from build123d import *

# Parameters (mm, degrees)
SKETCH1_R                = 1.75
BOSS_EXTRUDE1_DEPTH      = 3
BOSS_EXTRUDE2_DEPTH      = 15
BOSS_EXTRUDE3_REACH      = 34.671
BOSS_EXTRUDE3_END_RADIUS = 91.49157749
SKETCH4_R                = 1.75
CUT_EXTRUDE1_DEPTH       = 31.604747935


with BuildPart() as part:
    # Sketch1 → Boss-Extrude1 (new body)
    with BuildSketch(Plane.XY):
        with BuildLine():
            Line((0.117990197, 5), (14.645149272, 5))
            ThreePointArc((14.645149272, 5), (15.76191903, 15.092961754), (17.99029172, 25))
            Line((17.99029172, 25), (2.99029172, 25))
            ThreePointArc((2.99029172, 25), (1.076516113, 15.068594129), (0.117990197, 5))
        make_face()
        with Locations((3.988971184, 10)):
            Circle(SKETCH1_R, mode=Mode.SUBTRACT)
        with Locations((5.276368215, 19)):
            Circle(SKETCH1_R, mode=Mode.SUBTRACT)
    extrude(amount=BOSS_EXTRUDE1_DEPTH)

    # Sketch2 → Boss-Extrude2 (add)
    with BuildSketch(Plane.XY.offset(3)):
        with BuildLine():
            Line((0.117990197, 5), (14.645149272, 5))
            ThreePointArc((14.645149272, 5), (14.739672725, 6.500878193), (14.858852588, 8))
            Line((14.858852588, 8), (0.302317906, 8))
            ThreePointArc((0.302317906, 8), (0.199520295, 6.500653365), (0.117990197, 5))
        make_face()
    extrude(amount=BOSS_EXTRUDE2_DEPTH)

    # Boss-Extrude3: up to this cylinder (the profile starts outside it)
    boss_extrude3_end = Plane(origin=(106, 0, 8), z_dir=(0, 0, -1)) * Cylinder(BOSS_EXTRUDE3_END_RADIUS, 253.32515498, mode=Mode.PRIVATE)
    # Sketch3 → Boss-Extrude3 (add, up to the surface)
    with BuildSketch(Plane(origin=(11, 0, 0), x_dir=(0, 0, -1), z_dir=(1, 0, 0)), mode=Mode.PRIVATE) as boss_extrude3_sk1:
        Polygon((-18, 8), (-3, 25), (-3, 8), align=None)
    boss_extrude3_tool1 = extrude(boss_extrude3_sk1.sketch, amount=BOSS_EXTRUDE3_REACH, mode=Mode.PRIVATE) - boss_extrude3_end
    add(boss_extrude3_tool1.solids().sort_by_distance((11, 13.666667, 8))[0])

    # Sketch4 → Cut-Extrude1 (cut, through all)
    with BuildSketch(Plane(origin=(0, 8, 0), x_dir=(1, 0, 0), z_dir=(0, 1, 0))):
        with Locations(Location((5, -12.5, 0), (0, 0, 270))):
            Circle(SKETCH4_R)
    extrude(amount=-CUT_EXTRUDE1_DEPTH, mode=Mode.SUBTRACT)


solid = part.part
Verification items for the finished model (mm, model axes). A direction names the side the tool comes from. Coordinates: 2 decimals unless noted, no trailing zeros. Write each loop counter-clockwise with the first axis right and the second up, starting at its lowest first coordinate (ties: lowest second). Pieces come first, ordered by that corner, then holes. Notation, with made-up numbers: M 60,55.25 L 113,55.25 A28 cw 113,86.25 Z; hole C 11,52.5 d8. An arc over 180 degrees is marked long. Use CSV: the item, a comma, the result in double quotes.
Q1. Mould release check, pull along X, two halves, no side actions. Record for faces 1 (the flat face through (7, 7, 18)), 2 (the flat face through (11, 13, 7)), 3 (the cylindrical face through (3.761, 11.735, 1.479)): pulls with the +X half, pulls with the -X half, needs draft (parallel to the pull), parting line crosses it, or undercut.
Computed values:
face 1,"needs draft"
face 2,"pulls with the -X half"
face 3,"undercut"
Q2. Section check D-D, the plane x = 5. Enter the section's corners in (y, z).
Computed values:
outline,"M 5,0 L 8.57,0 L 8.57,3 L 8,3 L 8,10.75 L 5,10.75 Z; M 5,14.25 L 8,14.25 L 8,18 L 5,18 Z; M 11.43,0 L 17.27,0 L 17.27,3 L 11.43,3 Z; M 20.73,0 L 25,0 L 25,3 L 20.73,3 Z"
Q3. Section check A-A, the plane z = 11.5. Enter the section's corners in (x, y), and give its area (3 significant figures).
Computed values:
outline,"M 0.12,5 L 3.56,5 L 3.56,8 L 0.3,8 A106 ccw Z; M 6.44,5 L 14.65,5 A91.49 cw 14.86,8 A91.49 cw 15.81,15.37 L 11,15.37 L 11,8 L 6.44,8 Z"
area,"66.6 mm²"
Q4. Thickness scan on line 1 along Z through (x, y) = (9, 10.25); line 2 along X through (y, z) = (6.7, 12.5); line 3 along X through (y, z) = (6, 12.5). Record the ranges inside material, lowest first. Write a range as [from, to].
Computed values:
line 1,"[0, 3]"
line 2,"[0.21, 3.25], [6.75, 14.75]"
line 3,"[0.17, 3.25], [6.75, 14.71]"
Q5. Set-up check for faces 4 (the cylindrical face through (5.049, 20.735, 1.479)), 5 (the flat face through (7, 17, 3)): record each of +Z, -Z, +X, -X, +Y, -Y from which the full face is reachable in a straight line by a thin tool's end or side.
Computed values:
face 4,"+Z, -Z"
face 5,"+Z, -X, +Y"
Q6. Section check B-B, the plane y = 20. Enter the section's corners in (x, z).
Computed values:
outline,"M 1.9,0 L 3.84,0 L 3.84,3 L 1.9,3 Z; M 6.71,0 L 16.72,0 L 16.72,7.41 L 11,7.41 L 11,3 L 6.71,3 Z"
Q7. Section check C-C, the plane x = 12.75. Enter the section's corners in (y, z), and give its area (4 significant figures).
Computed values:
outline,"M 5,0 L 25,0 L 25,3 L 8,18 L 5,18 Z"
area,"232.5 mm²"
Q8. Go/stop test with flat-tipped pins: P1, Ø4.5, axis at y = 15.5, z = 12.5, coming from the -X side; P2, Ø3, axis at y = 22, z = 8.5, coming from the +X side; P3, Ø10, axis at y = 8.5, z = 8.5, coming from the +X side; P4, Ø5.5, axis at x = 8, z = 7, coming from the +Y side. Record where each tip stops, or that it passes through.
Computed values:
P1,"x = 11"
P2,"through"
P3,"x = 15.51"
P4,"y = 8"
